Verification items for the finished model (mm, model axes). A direction names the side the tool comes from. Round coordinates to 2 decimals unless told otherwise and drop trailing zeros. Write each loop counter-clockwise with the first axis right and the second up, starting at its lowest first coordinate (ties: lowest second). Pieces come first, ordered by that corner, then holes. Notation, with made-up numbers: M 39.25,-39.5 L 47.25,-39.5 A33 cw 47.25,-2.5 Z; hole C 56,21 d11. An arc over 180 degrees is marked long. Answer in a Markdown table with one row per item. Add a question column.
1. Draft check along Y on faces 1 (the flat face through (-5, -9, 34)), 2 (the cylindrical face through (46.737, 14.718, 14.79)), 3 (the flat face through (-37, 0, 18)). Enter one of: pulls with the +Y half, pulls with the -Y half, needs draft (parallel to the pull), parting line crosses it, or undercut.
2. Go/stop test with flat-tipped pins: pin 1 Ø5 at (x, y) = (22.5, 33) entering from +Z; pin 2 Ø4.5 at (x, y) = (-30, -0.05) entering from -Z; pin 3 Ø2 at (y, z) = (-6, 16.5) entering from +X. Record where each tip stops, or that it passes through.
3. Sectioned sample at C-C on x = 23.5. Record the cut outline in (y, z).
4. Set-up check for faces 4 (the cylindrical face through (-40.3, -20.9, 17.7)), 5 (the cylindrical face through (13.354, -27.798, 9.86)): record each of +Z, -Z, +X, -X, +Y, -Y from which the full face is reachable in a straight line by a thin tool's end or side.
5. Sectioned sample at D-D on y = -33.5. Record the cut outline in (x, z).
6. Sectioned sample at B-B on z = 43.5. Record the cut outline in (x, y).
7. Sectioned sample at A-A on z = 18. Count the separate pieces of the cut face and the enclosed holes in it, plus the area to 3 significant figures.
8. Material ranges on probe 1 along X at (y, z) = (20.5, 25); probe 2 along Z at (x, y) = (-42, 0); probe 3 along Z at (x, y) = (-9, -30), recorded low to high.
```python
from build123d import *

# Parameters (mm, degrees)
ESQUISSE1_R                  = 49
BASE_EXTRUSION_DEPTH         = 30
ESQUISSE20_R                 = 3
ENL_V_MAT_EXTRU_4_DEPTH      = 12
ESQUISSE3_R                  = 10
BOSS_EXTRU_1_DEPTH           = 46
ESQUISSE11_R                 = 3
ENL_V_MAT_EXTRU_3_DEPTH      = 31.0000001
R_P_TITION_CIRCULAIRE1_COUNT = 6
R_P_TITION_CIRCULAIRE3_COUNT = 2
R_P_TITION_CIRCULAIRE3_ANGLE = 135
R_P_TITION_CIRCULAIRE4_COUNT = 3


with BuildPart() as part:
    # Esquisse1 → Base-Extrusion (new body)
    with BuildSketch(Plane.XY):
        Circle(ESQUISSE1_R)
    extrude(amount=BASE_EXTRUSION_DEPTH)

    # Esquisse2 → Boss.-Révol.1 (revolve)
    with BuildSketch(Plane(origin=(0, 0, 0), x_dir=(0, 0, -1), z_dir=(1, 0, 0))):
        Polygon((-30, 0), (-30, 17.5), (-34, 13.5), (-34, 0), align=None)
    revolve(axis=Axis((0, 0, 38.858858859), (0, 0, -1)))

    # Esquisse20 → Enlèv. mat.-Extru.4 (cut)
    with BuildSketch(Plane(origin=(-49, 0, 15), x_dir=(0, 1, 0), z_dir=(-1, 0, 0))):
        with Locations((0, -3)):
            Circle(ESQUISSE20_R)
    extrude(amount=-ENL_V_MAT_EXTRU_4_DEPTH, mode=Mode.SUBTRACT)

    # Esquisse3 → Boss.-Extru.1 (add)
    with BuildSketch(Plane.XY.offset(34)):
        Circle(ESQUISSE3_R)
    extrude(amount=BOSS_EXTRU_1_DEPTH)

    # Esquisse11 → Enlèv. mat.-Extru.3 (cut, through all)
    with BuildSketch(Plane.XY.offset(30)):
        with Locations((-22, -38.105117767)):
            Circle(ESQUISSE11_R)
    extrude(amount=-ENL_V_MAT_EXTRU_3_DEPTH, mode=Mode.SUBTRACT)

    # Esquisse12 → Perçage2 (revolve, cut)
    with BuildSketch(Plane(origin=(0, -44, 30), x_dir=(0, -1, 0), z_dir=(1, 0, 0))):
        Polygon((0, 0), (0, 26.47511282), (2.455, 25), (2.455, 0), align=None)
    per_age2 = revolve(axis=Axis((0, -44, 34.244199587), (0, 0, -1)), mode=Mode.SUBTRACT)

    # Répétition circulaire1: Perçage2 ×6 about axis
    r_p_tition_circulaire1_axis = Axis((0, 0, 0), (0, 0, 1))
    for i in range(1, R_P_TITION_CIRCULAIRE1_COUNT):
        add(per_age2.rotate(r_p_tition_circulaire1_axis, i * 360 / R_P_TITION_CIRCULAIRE1_COUNT), mode=Mode.SUBTRACT)

    # Esquisse16 → Perçage4 (revolve, cut)
    with BuildSketch(Plane(origin=(-21.242014496, 21.184353192, 0), x_dir=(0, 1, 0), z_dir=(1, 0, 0))):
        Polygon((0, 0), (0, 21.802581857), (3, 20), (3, 0), align=None)
    per_age4 = revolve(axis=Axis((-21.242014496, 21.184353192, -6.35), (0, 0, 1)), mode=Mode.SUBTRACT)

    # Répétition circulaire3: Perçage4 ×2 about axis
    r_p_tition_circulaire3_axis = Axis((0, 0, 0), (0, 0, -1))
    for i in range(1, R_P_TITION_CIRCULAIRE3_COUNT):
        add(per_age4.rotate(r_p_tition_circulaire3_axis, i * R_P_TITION_CIRCULAIRE3_ANGLE / (R_P_TITION_CIRCULAIRE3_COUNT - 1)), mode=Mode.SUBTRACT)

    # Esquisse18 → Perçage5 (revolve, cut)
    with BuildSketch(Plane(origin=(-30, -0.050785262, 0), x_dir=(0, 1, 0), z_dir=(1, 0, 0))):
        Polygon((0, 0), (0, 21.502151548), (2.5, 20), (2.5, 0), align=None)
    per_age5 = revolve(axis=Axis((-30, -0.050785262, -6.35), (0, 0, 1)), mode=Mode.SUBTRACT)

    # Répétition circulaire4: Perçage5 ×3 about axis
    r_p_tition_circulaire4_axis = Axis((0, 0, 0), (0, 0, 1))
    for i in range(1, R_P_TITION_CIRCULAIRE4_COUNT):
        add(per_age5.rotate(r_p_tition_circulaire4_axis, i * 360 / R_P_TITION_CIRCULAIRE4_COUNT), mode=Mode.SUBTRACT)


solid = part.part
```
Geometry check:
| question | item | result |
|---|---|---|
| 1 | face 1 | needs draft |
| 1 | face 2 | parting line crosses it |
| 1 | face 3 | undercut |
| 2 | pin 1 | stops at z = 30 |
| 2 | pin 2 | stops at z = 20.15 |
| 2 | pin 3 | stops at x = 48.74 |
| 3 | outline | M -43,0 L 43,0 L 43,30 L -43,30 Z |
| 4 | face 4 | +Z |
| 4 | face 5 | -Z |
| 5 | outline | M -35.76,0 L 35.76,0 L 35.76,30 L -35.76,30 Z |
| 6 | outline | C 0,0 d20 |
| 7 | separate pieces | 1 |
| 7 | enclosed holes | 12 |
| 7 | area | 7,210 mm2 |
| 8 | probe 1 | x = -44.51 to -40.05, -36.16 to 36.16, 40.05 to 44.51 |
| 8 | probe 2 | z = 0 to 15, 21 to 30 |
| 8 | probe 3 | z = 0 to 30 |
